CAD build for the part. Positions are in the model's coordinates, mm. A direction names the side the tool comes from. Round coordinates to 2 decimals unless told otherwise and drop trailing zeros. Loops run counter-clockwise (first coordinate to the right, second up) from the corner with the lowest first, then second, coordinate; pieces in that order, holes last.
from build123d import *

# Parameters (mm, degrees)
BOSS_EXTRUDE1_DEPTH = 125
CUT_EXTRUDE1_DEPTH  = 250
SKETCH2_R           = 28.1
CUT_EXTRUDE2_DEPTH  = 150


with BuildPart() as part:
    # Sketch1 → Boss-Extrude1 (new, symmetric)
    with BuildSketch(Plane.XY):
        Polygon((0, 0), (0, -260), (400, -260), (400, -160), (100, -25), (100, 0), align=None)
    extrude(amount=BOSS_EXTRUDE1_DEPTH, both=True)

    # 3DSketch1 → Cut-Extrude1 (cut, along a direction that is not the sketch's normal)
    with BuildSketch(Plane(origin=(150, -47.5, 125), x_dir=(0.7367094686837573, -0.3315192609076908, -0.5893675749470058), z_dir=(-0.6052160263325688, -0.7120188545089043, -0.3560094272544522))):
        Polygon((0, 0), (339.346799012, 0), (254.625210114, 206.935382123), align=None)
    extrude(amount=-CUT_EXTRUDE1_DEPTH, dir=(0, -1, 0), mode=Mode.SUBTRACT)

    # Sketch2 → Cut-Extrude2 (cut)
    with BuildSketch(Plane(origin=(0, 0, 0), x_dir=(1, 0, 0), z_dir=(0, 1, 0))):
        with Locations(Location((50, 0, 0), (0, 0, 180))):
            Circle(SKETCH2_R)
    extrude(amount=-CUT_EXTRUDE2_DEPTH, mode=Mode.SUBTRACT)


solid = part.part
Item 1: Cut at B-B (z = 52). List the corners of the cut face in (x, y).
Verdict:
outline: (0, -260) - (400, -260) - (400, -223.5) - (241.25, -88.56) - (100, -25) - (100, 0) - (0, 0) - close
Item 2: Cut at C-C (x = 50). List the corners of the cut face in (y, z), plus the area to 3 significant figures.
Verdict:
outline: (-260, -125) - (0, -125) - (0, -28.1) - (-150, -28.1) - (-150, 28.1) - (0, 28.1) - (0, 125) - (-260, 125) - close
area: 56,600 mm2
Item 3: Wall check: L1, parallel to Z at x = 49.5, y = -99; L2, parallel to X at y = -11.5, z = 95; L3, parallel to Y at x = 52.5, z = 23. Give the ranges that are in metal, low to high.
Verdict:
L1: z = -125 to -28.1, 28.1 to 125
L2: x = 0 to 100
L3: y = -260 to -150
Item 4: Mould opens along X. For faces 1 (the flat face through (197, -260, 2)), 2 (the flat face through (50, -150, 0)), 3 (the flat face through (218.767, -78.445, -26.028)) say: released by +X, released by -X, zero draft, split by the parting line, or undercut.
Verdict:
face 1: zero draft
face 2: undercut
face 3: released by +X
Item 5: Flat gauge pins, fed straight in: P1, Ø20, axis at y = -7, z = -51, coming from the +X side; P2, Ø2, axis at x = 322.5, z = -16.5, coming from the +Y side (3 decimals); P3, Ø4, axis at y = -148, z = -40.5, coming from the +X side; P4, Ø10, axis at x = 51, z = -75, coming from the +Y side. Where does each tip first touch, or does it go through?
Verdict:
P1: stops at x = 100
P2: stops at y = -124.675
P3: stops at x = 368.22
P4: stops at y = 0
Item 6: 3-axis set-ups, long thin cutter, end or side, ignore diameter. For faces 4 (the flat face through (100, -13, 2)), 5 (the flat face through (153, -157, -125)), 6 (the cylindrical face through (24.04, -73.95, -10.76)): which of +Z, -Z, +X, -X, +Y, -Y reach the whole face in a straight line?
Verdict:
face 4: +Z, -Z, +X, +Y
face 5: -Z, +X, -X, +Y, -Y
face 6: +Y
Item 7: Cut at A-A (y = -90). List the corners of the cut face in (x, z), plus the area to 3 significant figures.
Verdict:
outline: (0, -125) - (244.44, -125) - (244.44, 49.44) - (200, 125) - (0, 125) - close; hole circle Ø56.2 at (50, 0)
area: 57,000 mm2
Item 8: Cut at D-D (y = -190.5). List the corners of the cut face in (x, z), plus the area to 3 significant figures.
Verdict:
outline: (0, -125) - (400, -125) - (400, -14) - (318.24, 125) - (0, 125) - close
area: 94,300 mm2
